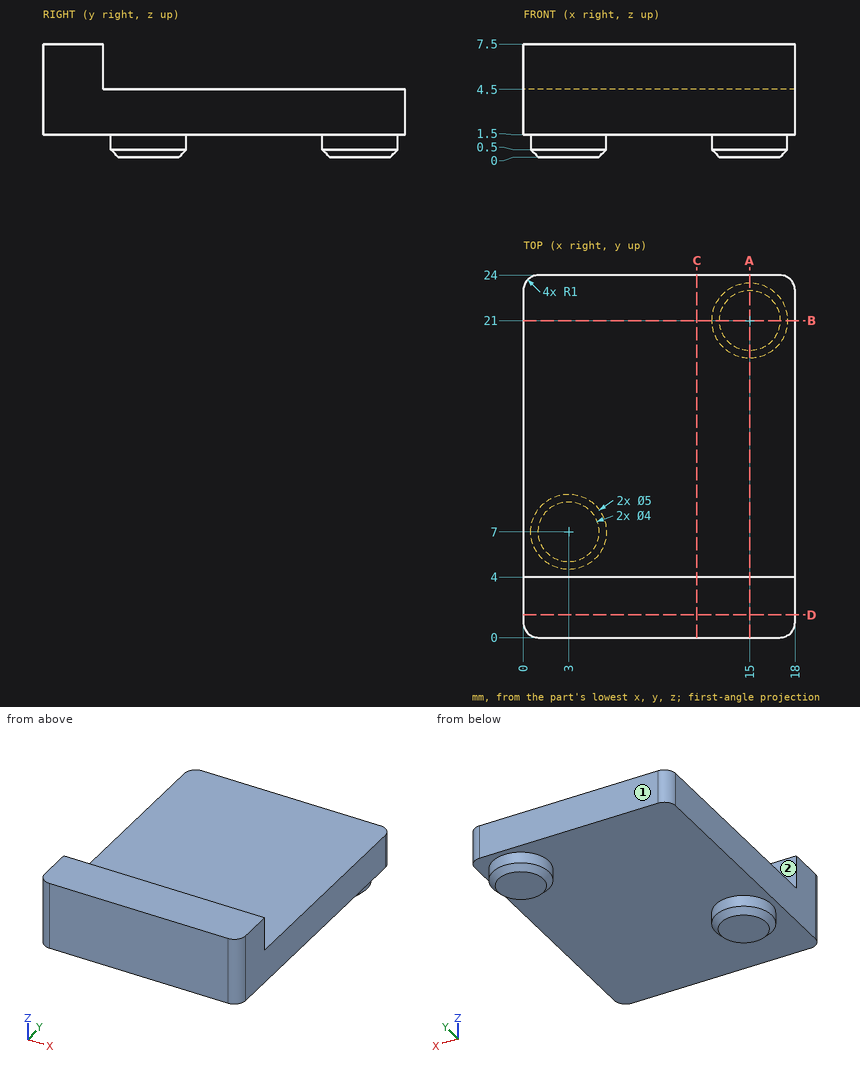
For this review, use the dimensioned drawing (mm, ordinates from the lowest corner) and the shaded views. A direction names the side the tool comes from. Give positions to 0.01 mm unless a question says otherwise; leave off trailing zeros. Write each loop counter-clockwise with the first axis right and the second up, starting at its lowest first coordinate (ties: lowest second). Pieces come first, ordered by that corner, then holes.
(1) To check wall thickness, follow L1, parallel to Z at x = 5.75, y = 22.5; L2, parallel to Z at x = 15.25, y = 2.75; L3, parallel to Y at x = 8.25, z = 7.25. State the ranges of each line that lie inside material, in increasing order.
(2) Consider section D-D, the plane y = 1.5. Give the boundary of the cut face in (x, z).
(3) Consider section C-C, the plane x = 11.5. Give the boundary of the cut face in (y, z), and give its area (3 significant figures).
(4) Consider section A-A, the plane x = 15. Give the boundary of the cut face in (y, z).
(5) Consider section B-B, the plane y = 21. Give the boundary of the cut face in (x, z).
(6) For P1, Ø1.5, axis at x = 6, z = 5.5, coming from the +Y side; P2, Ø1.5, axis at x = 10.5, y = 9.5, coming from the -Z side, all flat-tipped, find the tip position at first contact; note any pin that passes through.
(7) Tool access review of the marked faces 1 and 2: name each direction out of +Z, -Z, +X, -X, +Y, -Y from which nothing blocks a thin tool from reaching the whole face with its end or side.
Returned:
1. L1: z = 1.5 to 4.5
1. L2: z = 1.5 to 7.5
1. L3: y = 0 to 4
2. outline: (0, 1.5) - (18, 1.5) - (18, 7.5) - (0, 7.5) - close
3. outline: (0, 1.5) - (24, 1.5) - (24, 4.5) - (4, 4.5) - (4, 7.5) - (0, 7.5) - close
3. area: 84.0 mm2
4. outline: (0, 1.5) - (18.5, 1.5) - (18.5, 0.5) - (19, 0) - (23, 0) - (23.5, 0.5) - (23.5, 1.5) - (24, 1.5) - (24, 4.5) - (4, 4.5) - (4, 7.5) - (0, 7.5) - close
5. outline: (0, 1.5) - (12.5, 1.5) - (12.5, 0.5) - (13, 0) - (17, 0) - (17.5, 0.5) - (17.5, 1.5) - (18, 1.5) - (18, 4.5) - (0, 4.5) - close
6. P1: stops at y = 4
6. P2: stops at z = 1.5
7. face 1: +Z, -Z, +X, -X, +Y
7. face 2: +Z, +X, -X, +Y
